Part print with two shaded views. Sizes in mm from the minimum x, y, z corner. A direction names the side the tool comes from. Coordinates: 2 decimals unless noted, no trailing zeros. Loops run counter-clockwise (first coordinate to the right, second up) from the corner with the lowest first, then second, coordinate; pieces in that order, holes last.
Item 1: Mould opens along X. For the marked faces 1, 2 and 3 say: released by +X, released by -X, zero draft, split by the parting line, or undercut.
Item 2: Cut at A-A (y = 7.5). List the corners of the cut face in (x, z), and give its area (3 significant figures).
Item 3: Cut at C-C (z = 12). List the corners of the cut face in (x, y), and give its area (3 significant figures).
Item 4: Cut at D-D (z = 7.25). List the corners of the cut face in (x, y).
Item 5: 3-axis set-ups, long thin cutter, end or side, ignore diameter. For the marked faces 4 and 5: which of +Z, -Z, +X, -X, +Y, -Y reach the whole face in a straight line?
Item 6: Drill centre lines: line 1 along Y through (x, z) = (7.5, 1.55); line 2 along Y through (x, z) = (7.5, 9.5); line 3 along Z through (x, y) = (12.5, 9). Where is each one in solid material? Low to high.
Item 7: Flat gauge pins, fed straight in: pin 1 (5 mm diameter, centred on x = 7.5, y = 7.5, fed in from -Z); pin 2 (1.5 mm diameter, centred on y = 9.5, z = 2.5, fed in from +X); pin 3 (3 mm diameter, centred on x = 9.5, z = 8.5, fed in from +Y). Where does each tip first touch, or does it go through?
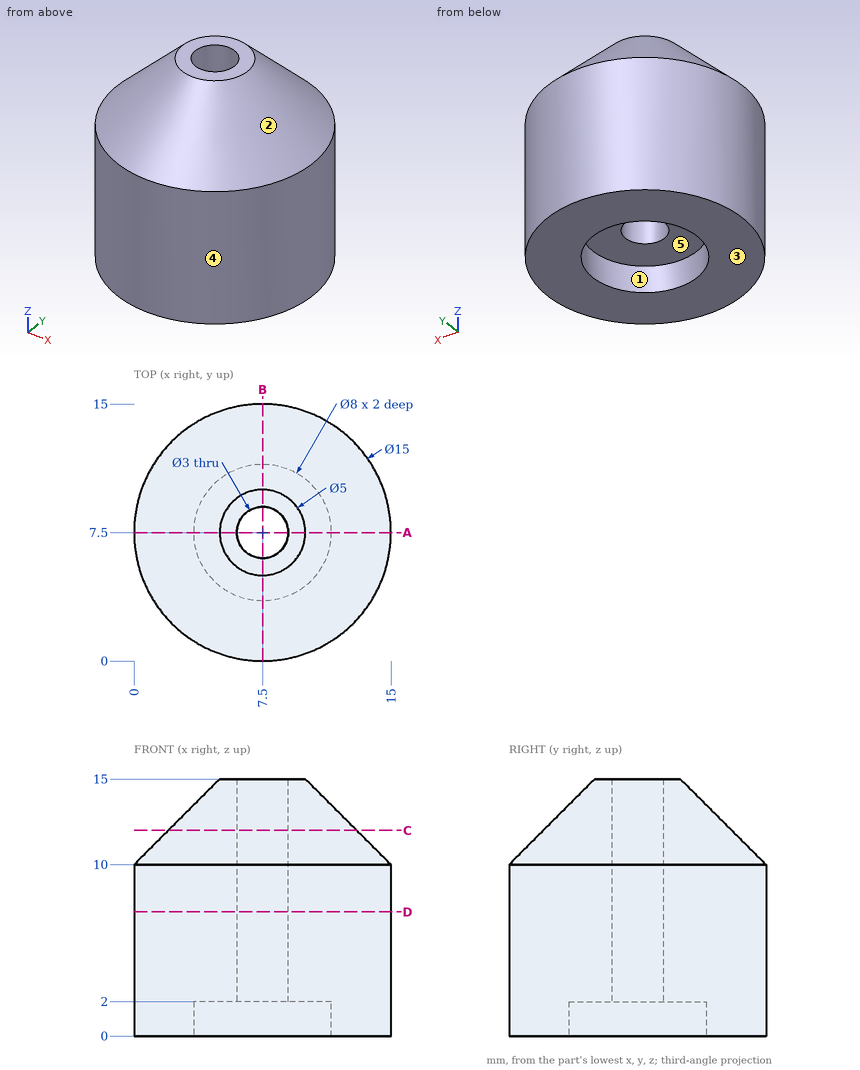
Filled sheet:
1. face 1: undercut
1. face 2: split by the parting line
1. face 3: zero draft
2. outline: (0, 0) - (3.5, 0) - (3.5, 2) - (6, 2) - (6, 15) - (5, 15) - (0, 10) - close; (9, 2) - (11.5, 2) - (11.5, 0) - (15, 0) - (15, 10) - (10, 15) - (9, 15) - close
2. area: 145 mm2
3. outline: circle Ø11 at (7.5, 7.5); hole circle Ø3 at (7.5, 7.5)
3. area: 88.0 mm2
4. outline: circle Ø15 at (7.5, 7.5); hole circle Ø3 at (7.5, 7.5)
5. face 4: +Z, -Z
5. face 5: -Z
6. line 1: y = 0 to 3.5, 11.5 to 15
6. line 2: y = 0 to 6, 9 to 15
6. line 3: z = 0 to 12.28
7. pin 1: stops at z = 2
7. pin 2: stops at x = 14.9
7. pin 3: stops at y = 14.98
